Source: three-view drawing plus pictorial views. Frame: mm from the lowest corner of the part. A direction names the side the tool comes from. Give positions to 0.01 mm unless a question says otherwise; leave off trailing zeros. Order: outer loops, then holes, each group sorted by start corner. A loop starts at its lowest first (then second) coordinate and runs counter-clockwise, first axis right, second up. Notation, with made-up numbers: M 77,-28.75 L 115,-28.75 A24 ccw 115,-10.75 Z; hole C 70.5,-34.5 d11. An arc over 180 degrees is marked long. Use CSV: the item, a comma, the result in double quotes. Start each with the question number.
Item 1: Section query B-B on x = 13.7. Return loops of the section in (y, z).
Item 2: Access query for the marked faces 1 and 2. Directions: +Z, -Z, +X, -X, +Y, -Y. A direction counts if a zero-diameter tool reaches every point of the face in a straight line with its end or side. Return the directions, or none.
Item 3: First-contact query: pin 1 (7 mm diameter, centred on x = 28.5, y = 11.5, fed in from +Z); pin 2 (6.5 mm diameter, centred on x = 28.7, y = 13.5, fed in from +Z). Flat tips, straight axial feed; report the tip coordinate or a pass-through.
Item 4: Section query C-C on z = 7. Return loops of the section in (x, y).
Item 5: Section query A-A on y = 13.5. Return loops of the section in (x, z).
Item 6: Section query D-D on x = 28.7. Return loops of the section in (y, z), and give its area (3 significant figures).
Item 7: Ray query, probe 1 along Z at (x, y) = (21.5, 17); probe 2 along X at (y, z) = (7.5, 5.5); probe 3 along Y at (x, z) = (19.5, 3.75). Return the intervals inside material, ascending. Write a range as from..to.
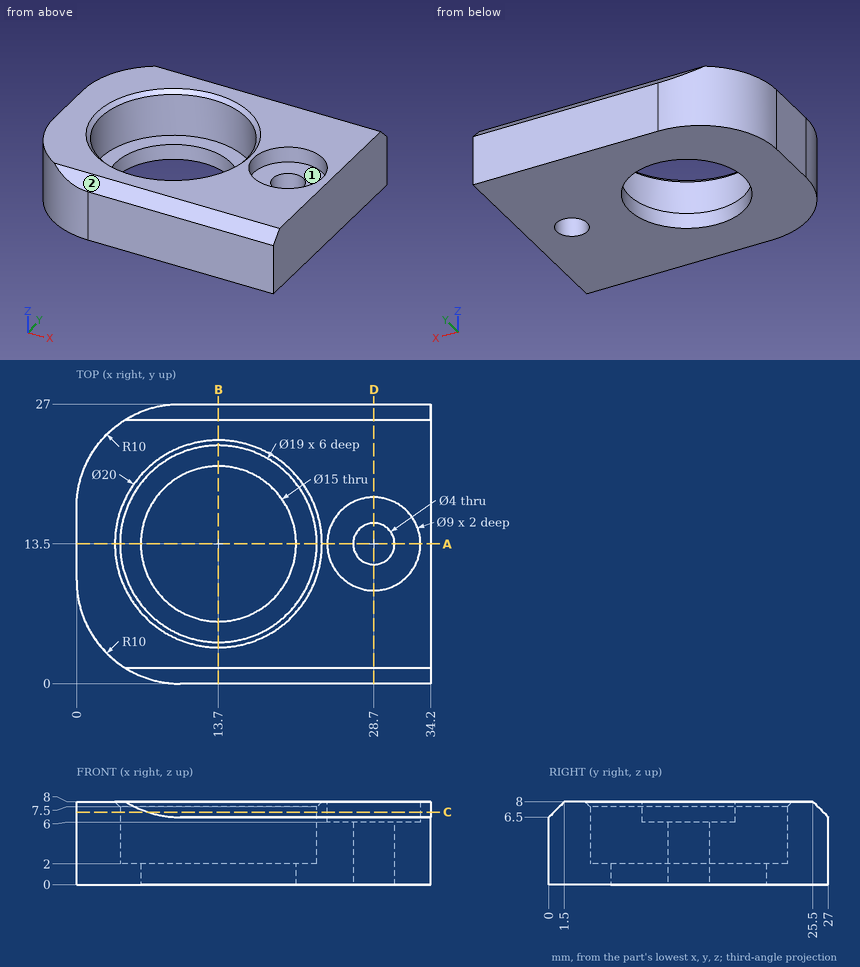
Verdict:
1,outline,"M 0,0 L 6,0 L 6,2 L 4,2 L 4,7.5 L 3.5,8 L 1.5,8 L 0,6.5 Z; M 21,0 L 27,0 L 27,6.5 L 25.5,8 L 23.5,8 L 23,7.5 L 23,2 L 21,2 Z"
2,face 1,"+Z"
2,face 2,"+Z, +X, -X, -Y"
3,pin 1,"z = 8"
3,pin 2,"z = 6"
4,outline,"M 0,10 A10 ccw 6.88,0.5 L 34.2,0.5 L 34.2,26.5 L 6.88,26.5 A10 ccw 0,17 Z; hole C 13.7,13.5 d19; hole C 28.7,13.5 d9"
5,outline,"M 0,0 L 6.2,0 L 6.2,2 L 4.2,2 L 4.2,7.5 L 3.7,8 L 0,8 Z; M 21.2,0 L 26.7,0 L 26.7,6 L 24.2,6 L 24.2,8 L 23.7,8 L 23.2,7.5 L 23.2,2 L 21.2,2 Z; M 30.7,0 L 34.2,0 L 34.2,8 L 33.2,8 L 33.2,6 L 30.7,6 Z"
6,outline,"M 0,0 L 11.5,0 L 11.5,6 L 9,6 L 9,8 L 1.5,8 L 0,6.5 Z; M 15.5,0 L 27,0 L 27,6.5 L 25.5,8 L 18,8 L 18,6 L 15.5,6 Z"
6,area,"172 mm2"
7,probe 1,"0..2"
7,probe 2,"0.32..6.33, 21.07..34.2"
7,probe 3,"0..5.98, 21.02..27"
